Could you check a few things on this model? Use its own coordinates, in mm. A direction names the side the tool comes from. Coordinates: 2 decimals unless noted, no trailing zeros. Loops run counter-clockwise (first coordinate to the right, second up) from the corner with the lowest first, then second, coordinate; pieces in that order, holes last.
Autodesk Inventor part; units mm, degrees
ref_plane "YZ Plane" through (0, 0, 0) normal (1, 0, 0) x (0, 1, 0)
ref_plane "XZ Plane" through (0, 0, 0) normal (0, 1, 0) x (-1, 0, 0)
ref_plane "XY Plane" through (0, 0, 0) normal (0, 0, 1) x (1, 0, 0)
sketch "Sketch1" plane through (0, 0, 0) normal (0, 0, 1) x (1, 0, 0)
  line L0 (5, 0) -> (5, 3)
  line L1 (5, 0) -> (40, 0)
  line L2 (40, 0) -> (40, 3)
  line L3 (5, 3) -> (40, 3)
  line L4 (0, 0) -> (5, 0)
  line L5 (5, 0) -> (5, 3)
  line L6 (0, 3) -> (5, 3)
  line L7 (0, 0) -> (0, 3)
  line L8 (0, -2) -> (0, 3)
  line L9 (0, 3) -> (-3, 3)
  line L10 (-3, -2) -> (-3, 3)
  line L11 (0, -2) -> (-3, -2)
  line L12 (0, -10) -> (-3, -10)
  line L13 (0, -10) -> (0, -2)
  line L14 (0, -2) -> (-3, -2)
  line L15 (-3, -10) -> (-3, -2)
  line L16 (0, -15) -> (0, -10)
  line L17 (0, -10) -> (-3, -10)
  line L18 (-3, -15) -> (-3, -10)
  line L19 (0, -15) -> (-3, -15)
  line L20 (45, -10) -> (45, -15)
  line L21 (45, -15) -> (48, -15)
  line L22 (48, -10) -> (48, -15)
  line L23 (45, -10) -> (48, -10)
  line L24 (45, -2) -> (45, -10)
  line L25 (45, -10) -> (48, -10)
  line L26 (48, -2) -> (48, -10)
  line L27 (45, -2) -> (48, -2)
  line L28 (45, 3) -> (45, -2)
  line L29 (45, -2) -> (48, -2)
  line L30 (48, 3) -> (48, -2)
  line L31 (45, 3) -> (48, 3)
  line L32 (40, 0) -> (45, 0)
  line L33 (45, 0) -> (45, 3)
  line L34 (40, 3) -> (45, 3)
  line L35 (40, 0) -> (40, 3)
  line L36 (0, -15) -> (45, -15)
extrude "Extrusion1" add sketch "Sketch1" along normal blind 3 contours L0 L3 L2 L1 | L1 L32 L28 L24 L20 L36 L16 L13 L8 L4 | L13 L12 L15 L11 | L27 L26 L23 L24
properties part number "SideFaceTopNM" material "Acrylic, Clear"
1) If I drill on L1, parallel to X at y = 0.25, z = 0.3; L2, parallel to Y at x = 1.5, z = 2.25; L3, parallel to X at y = -12, z = 2.45, over which ranges is the centre line in solid material (lowest first)?
2) Imagine slicing it at A-A on z = 1.7. List the corners of the cut face in (x, y) for me.
3) For faces 4 (the flat face through (45, -1, 1)), 5 (the flat face through (0, -1, 1)), 6 (the flat face through (45, -12, 1)), 7 (the flat face through (0, -13, 1)), 8 (the flat face through (48, -6, 1)), which set-ups out of +Z, -Z, +X, -X, +Y, -Y let a thin tool reach every point of the face, with its end or its side?
4) Imagine slicing it at B-B on y = -0.75. List the corners of the cut face in (x, z) for me.
5) We'd pull the mould along Y, two halves only. Please class faces 1 (the flat face through (40, 1, 1)), 2 (the flat face through (42, 0, 1)), 3 (the flat face through (-1, -10, 1)): released by +Y, released by -Y, zero draft, split by the parting line, or undercut.
6) Will these pins go through, and if not, where does the flat tip stop? pin 1 (0.9 mm diameter, centred on y = 1, z = 1, fed in from +X); pin 2 (1 mm diameter, centred on y = -0.5, z = 1.5, fed in from +X); pin 3 (0.9 mm diameter, centred on x = -1, z = 1.5, fed in from +Y).
Solved:
1. L1: x = 5 to 40
1. L2: y = -15 to 0
1. L3: x = 0 to 45
2. outline: (-3, -10) - (0, -10) - (0, -15) - (45, -15) - (45, -10) - (48, -10) - (48, -2) - (45, -2) - (45, 0) - (40, 0) - (40, 3) - (5, 3) - (5, 0) - (0, 0) - (0, -2) - (-3, -2) - close
3. face 4: +Z, -Z, +X, +Y
3. face 5: +Z, -Z, -X, +Y
3. face 6: +Z, -Z, +X, -Y
3. face 7: +Z, -Z, -X, -Y
3. face 8: +Z, -Z, +X, +Y, -Y
4. outline: (0, 0) - (45, 0) - (45, 3) - (0, 3) - close
5. face 1: zero draft
5. face 2: released by +Y
5. face 3: released by -Y
6. pin 1: stops at x = 40
6. pin 2: stops at x = 45
6. pin 3: stops at y = -2
